Input: part model. Units: mm. Frame: model coordinates. A direction names the side the tool comes from. Round coordinates to 2 decimals unless told otherwise and drop trailing zeros. Loops run counter-clockwise (first coordinate to the right, second up) from the corner with the lowest first, then second, coordinate; pieces in that order, holes last. Notation, with made-up numbers: (54.25, 81) -> (110.25, 81) arc R17 ccw to (110.25, 101) -> close; hole circle Ø5 at (65, 64). An arc over 180 degrees is marked (long way). One line per question, with ' | ' between items. Start each with the question number.
Q1. Material intervals for L1, parallel to Y at x = -2.5, z = -1.5; L2, parallel to Z at x = 10.5, y = -11.25, sorted ascending.
Q2. Cut plane A-A on z = -0.5. Return loops of the section in (x, y).
Q3. Contact query for flat-ended pins moving along their axis: P1, Ø3.5, axis at y = 3.5, z = -3.5, coming from the +X side; P2, Ø5, axis at y = 4, z = -3, coming from the -X side; P3, Ø3, axis at x = -1, y = -11, coming from the +Z side. Output: stop coordinate, or through.
Q4. Cut plane B-B on y = 0. Return loops of the section in (x, z).
Q5. Cut plane C-C on x = -6.75. Return loops of the section in (y, z).
Q6. Cut plane D-D on z = 1.75. Return loops of the section in (x, y).
Q7. Access query for faces 1 (the face through (0, 13, 0)), 2 (the face through (-12.5, 0, -2)), 3 (the face through (-13.25, 3, 2)). Directions: +Z, -Z, +X, -X, +Y, -Y. A direction counts if a zero-diameter tool reaches every point of the face in a straight line with its end or side. Return the directions, or none.
from build123d import *

# Parameters (mm, degrees)
SKETCH_1_W      = 28.5
SKETCH_1_H      = 28.5
EXTRUDE_1_DEPTH = 0.8
SKETCH_2_W      = 26.5
SKETCH_2_H      = 19.5
EXTRUDE_2_DEPTH = 3
EXTRUDE_START   = -3.8
EXTRUDE_3_DEPTH = 4.6


with BuildPart() as part:
    # Эскиз1 → Бобышка-Вытянуть1 (new body)
    with BuildSketch(Plane.XY):
        Rectangle(SKETCH_1_W, SKETCH_1_H)
    extrude(amount=EXTRUDE_1_DEPTH)

    # Эскиз2 → Бобышка-Вытянуть2 (add)
    with BuildSketch(Plane.XY.offset(0.8)):
        with Locations((0, 3)):
            Rectangle(SKETCH_2_W, SKETCH_2_H)
    extrude(amount=EXTRUDE_2_DEPTH)

    # Эскиз5 → Бобышка-Вытянуть3 (add)
    with BuildSketch(Plane.XY.offset(3.8).offset(EXTRUDE_START)):
        with BuildLine():
            Line((-8.5, -12.5), (8.5, -12.5))
            ThreePointArc((8.5, -12.5), (11.328427125, -11.328427125), (12.5, -8.5))
            Line((12.5, -8.5), (12.5, 8.5))
            ThreePointArc((12.5, 8.5), (11.328427125, 11.328427125), (8.5, 12.5))
            Line((8.5, 12.5), (-8.5, 12.5))
            ThreePointArc((-8.5, 12.5), (-11.328427125, 11.328427125), (-12.5, 8.5))
            Line((-12.5, 8.5), (-12.5, -8.5))
            ThreePointArc((-12.5, -8.5), (-11.328427125, -11.328427125), (-8.5, -12.5))
        make_face()
    extrude(amount=-EXTRUDE_3_DEPTH)


solid = part.part
Results:
1) L1: -12.5 to 12.5 | L2: -4.6 to 0.8
2) outline: (-12.5, -8.5) arc R4 ccw to (-8.5, -12.5) -> (8.5, -12.5) arc R4 ccw to (12.5, -8.5) -> (12.5, 8.5) arc R4 ccw to (8.5, 12.5) -> (-8.5, 12.5) arc R4 ccw to (-12.5, 8.5) -> close
3) P1: x = 12.5 | P2: x = -12.5 | P3: z = 0.8
4) outline: (-14.25, 0) -> (-12.5, 0) -> (-12.5, -4.6) -> (12.5, -4.6) -> (12.5, 0) -> (14.25, 0) -> (14.25, 0.8) -> (13.25, 0.8) -> (13.25, 3.8) -> (-13.25, 3.8) -> (-13.25, 0.8) -> (-14.25, 0.8) -> close
5) outline: (-14.25, 0) -> (-12.5, 0) -> (-12.5, -4.6) -> (12.5, -4.6) -> (12.5, 0) -> (14.25, 0) -> (14.25, 0.8) -> (12.75, 0.8) -> (12.75, 3.8) -> (-6.75, 3.8) -> (-6.75, 0.8) -> (-14.25, 0.8) -> close
6) outline: (-13.25, -6.75) -> (13.25, -6.75) -> (13.25, 12.75) -> (-13.25, 12.75) -> close
7) face 1: -Z | face 2: -Z, -X, +Y, -Y | face 3: +Z, -X, +Y, -Y
